Autodesk Inventor part; units mm, degrees
ref_plane "YZ Plane" through (0, 0, 0) normal (1, 0, 0) x (0, 1, 0)
ref_plane "XZ Plane" through (0, 0, 0) normal (0, 1, 0) x (-1, 0, 0)
ref_plane "XY Plane" through (0, 0, 0) normal (0, 0, 1) x (1, 0, 0)
sketch "Sketch1" plane through (0, 0, 0) normal (0, 0, 1) x (1, 0, 0)
  line L0 (3.175, 0) -> (53.975, 0)
  line L1 (57.15, 3.175) -> (57.15, 53.975)
  line L2 (53.975, 57.15) -> (3.175, 57.15)
  line L3 (0, 53.975) -> (0, 3.175)
  arc A0 (3.175, 57.15) -> (0, 53.975) centre (3.175, 53.975) ccw
  arc A1 (57.15, 53.975) -> (53.975, 57.15) centre (53.975, 53.975) ccw
  arc A2 (53.975, 0) -> (57.15, 3.175) centre (53.975, 3.175) ccw
  arc A3 (0, 3.175) -> (3.175, 0) centre (3.175, 3.175) ccw
  point P0 (0, 0)
  point P1 (57.15, 57.15)
  point P2 (57.15, 0)
  point P3 (0, 57.15)
  dimension "d0" = 57.15
  dimension "d1" = 57.15
  dimension "d2" = 3.175
extrude "Extrusion1" add sketch "Sketch1" along normal blind 6.35
sketch "Sketch2" plane through (0, 0, 6.35) normal (0, 0, 1) x (1, 0, 0)
  arc A0 (57.15, 53.975) -> (53.975, 57.15) centre (53.975, 53.975) ccw
  line L0 (3.175, 57.15) -> (53.975, 57.15)
  arc A1 (3.175, 57.15) -> (0, 53.975) centre (3.175, 53.975) ccw
  line L1 (0, 3.175) -> (0, 53.975)
  arc A2 (0, 3.175) -> (3.175, 0) centre (3.175, 3.175) ccw
  line L2 (53.975, 0) -> (3.175, 0)
  arc A3 (53.975, 0) -> (57.15, 3.175) centre (53.975, 3.175) ccw
  line L3 (57.15, 53.975) -> (57.15, 3.175)
  circle A4 centre (3.175, 53.975) radius 3.175
  circle A5 centre (53.975, 53.975) radius 3.175
  circle A6 centre (53.975, 3.175) radius 3.175
  circle A7 centre (3.175, 3.175) radius 3.175
  line L4 (6.35, 53.975) -> (6.35, 55.5498)
  line L5 (3.175, 50.8) -> (1.6002, 50.8)
  line L6 (50.8, 53.975) -> (50.8, 55.5498)
  line L7 (53.975, 50.8) -> (55.5498, 50.8)
  line L8 (53.975, 6.35) -> (55.5498, 6.35)
  line L9 (50.8, 3.175) -> (50.8, 1.6002)
  line L10 (6.35, 3.175) -> (6.35, 1.6002)
  line L11 (3.175, 6.35) -> (1.6002, 6.35)
  line L12 (7.9502, 57.15) -> (49.1998, 57.15)
  line L13 (57.15, 49.1998) -> (57.15, 7.9502)
  line L14 (49.1998, 0) -> (7.9502, 0)
  line L15 (0, 7.9502) -> (0, 49.1998)
  arc A8 (1.6002, 50.8) -> (0, 49.1998) centre (1.6002, 49.1998) ccw
  arc A9 (7.9502, 57.15) -> (6.35, 55.5498) centre (7.9502, 55.5498) ccw
  arc A10 (50.8, 55.5498) -> (49.1998, 57.15) centre (49.1998, 55.5498) ccw
  arc A11 (57.15, 49.1998) -> (55.5498, 50.8) centre (55.5498, 49.1998) ccw
  arc A12 (55.5498, 6.35) -> (57.15, 7.9502) centre (55.5498, 7.9502) ccw
  arc A13 (49.1998, 0) -> (50.8, 1.6002) centre (49.1998, 1.6002) ccw
  arc A14 (6.35, 1.6002) -> (7.9502, 0) centre (7.9502, 1.6002) ccw
  arc A15 (0, 7.9502) -> (1.6002, 6.35) centre (1.6002, 7.9502) ccw
  point P0 (0, 0)
  point P1 (6.35, 57.15)
  point P2 (0, 50.8)
  point P3 (50.8, 57.15)
  point P4 (57.15, 50.8)
  point P5 (57.15, 6.35)
  point P6 (50.8, 0)
  point P7 (6.35, 0)
  point P8 (0, 6.35)
  dimension "d5" = 1.6002
extrude "Extrusion2" add sketch "Sketch2" along normal blind 69.85 contours L3 A12 L8 A6 L9 A13 L2 A14 L10 A7 L11 A15 L1 A8 L5 A4 L4 A9 L0 A10 L6 A5 L7 A11
sketch "Sketch3" plane through (0, 0, 0) normal (0, 0, -1) x (-1, 0, 0)
  arc A0 (-53.975, 57.15) -> (-57.15, 53.975) centre (-53.975, 53.975) ccw
  arc A1 (-57.15, 3.175) -> (-53.975, 0) centre (-53.975, 3.175) ccw
  arc A2 (-3.175, 0) -> (0, 3.175) centre (-3.175, 3.175) ccw
  arc A3 (0, 53.975) -> (-3.175, 57.15) centre (-3.175, 53.975) ccw
  circle A4 centre (-53.975, 53.975) radius 1.5875
  circle A5 centre (-3.175, 3.175) radius 1.5875
  circle A6 centre (-53.975, 3.175) radius 1.5875
  point P0 (0, 0)
  dimension "d8" = 3.175
  dimension "d10" = 3.175
  dimension "d11" = 3.175
hole "Hole1" at (53.975, 53.975, 0) at (3.175, 53.975, 0) at (3.175, 3.175, 0) at (53.975, 3.175, 0) direction (0, 0, 1) diameter 3.175 depth 25.4 tip angle 118
sketch "Sketch4" plane through (0, 0, 0) normal (0, 0, -1) x (-1, 0, 0)
  circle A0 centre (-28.575, 28.575) radius 3.175
  point P0 (0, 0)
  dimension "d19" = 6.35
extrude "Extrusion3" add sketch "Sketch4" along normal blind 25.4
properties part number "nema 23 frame size servo"
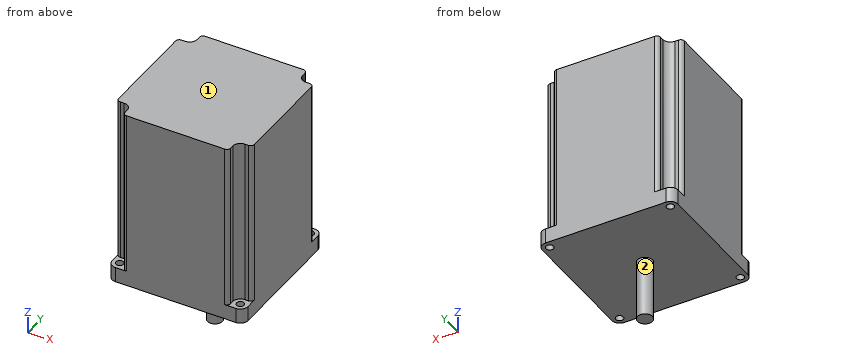
For this review, take the finished solid that the model builds, in its own axes (mm). Face numbers are marked on the shaded views. A direction names the side the tool comes from. Give positions to 0.01 mm unless a question says otherwise; leave off trailing zeros. Loops run counter-clockwise (first coordinate to the right, second up) from the corner with the lowest first, then second, coordinate; pieces in that order, holes last.
Item 1: Insertion check: pin 1 (0.8 mm diameter, centred on y = 2.5, z = 32.5, fed in from -X); pin 2 (1.3 mm diameter, centred on x = 2, z = 39.5, fed in from +Y); pin 3 (0.8 mm diameter, centred on x = 2.5, z = 51.5, fed in from -Y); pin 4 (2.5 mm diameter, centred on x = 53.975, y = 53.975, fed in from +Z). Each pin has a flat end and moves straight along its axis. Give the tip position at first contact, or say it passes through.
Item 2: Take a section at B-B, the plane y = 39. State the section outline as (x, z) points, and give its area (3 significant figures).
Item 3: Take a section at D-D, the plane x = 27.5. State the section outline as (y, z) points.
Item 4: Take a section at A-A, the plane z = 22. State the section outline as (x, y) points (3 decimals).
Item 5: For line 1 along Y through (x, z) = (4, 5); line 2 along Z through (x, y) = (6, 34); line 3 along X through (y, z) = (3, 16.5), list the stretches that pass through material, from the lowest coordinate up.
Item 6: Tool access review of the marked faces 1 and 2: name each direction out of +Z, -Z, +X, -X, +Y, -Y from which nothing blocks a thin tool from reaching the whole face with its end or side.
Calculated:
1. pin 1: stops at x = 6.35
1. pin 2: stops at y = 50.8
1. pin 3: stops at y = 6.35
1. pin 4: passes through
2. outline: (0, 0) - (57.15, 0) - (57.15, 76.2) - (0, 76.2) - close
2. area: 4,350 mm2
3. outline: (0, 0) - (25.59, 0) - (25.59, -25.4) - (31.56, -25.4) - (31.56, 0) - (57.15, 0) - (57.15, 76.2) - (0, 76.2) - close
4. outline: (0, 7.95) arc R1.6 ccw to (1.6, 6.35) - (3.175, 6.35) arc R3.175 cw to (6.35, 3.175) - (6.35, 1.6) arc R1.6 ccw to (7.95, 0) - (49.2, 0) arc R1.6 ccw to (50.8, 1.6) - (50.8, 3.175) arc R3.175 cw to (53.975, 6.35) - (55.55, 6.35) arc R1.6 ccw to (57.15, 7.95) - (57.15, 49.2) arc R1.6 ccw to (55.55, 50.8) - (53.975, 50.8) arc R3.175 cw to (50.8, 53.975) - (50.8, 55.55) arc R1.6 ccw to (49.2, 57.15) - (7.95, 57.15) arc R1.6 ccw to (6.35, 55.55) - (6.35, 53.975) arc R3.175 cw to (3.175, 50.8) - (1.6, 50.8) arc R1.6 ccw to (0, 49.2) - close
5. line 1: y = 0 to 1.82, 4.53 to 52.62, 55.33 to 57.15
5. line 2: z = 0 to 76.2
5. line 3: x = 6.35 to 50.8
6. face 1: +Z, +X, -X, +Y, -Y
6. face 2: -Z
